Input: part model. Units: mm. Frame: model coordinates. A direction names the side the tool comes from. Give positions to 0.01 mm unless a question says otherwise; leave off trailing zeros. Order: outer loops, then holes, each group sorted by start corner. A loop starts at its lowest first (then second) coordinate and runs counter-clockwise, first axis right, second up. Notation, with made-up numbers: (62.5, 31) - (116.5, 31) arc R12 ccw to (116.5, 52) - close; hole circle Ø9 at (78.25, 5.25). An arc over 180 degrees is marked (long way). Answer in a Markdown table with one row per item. Add a question column.
1. Section query D-D on y = 48.5. Return loops of the section in (x, z).
2. Section query C-C on z = 0. Return loops of the section in (x, y).
3. Mould query, pull axis Y, two halves, no side actions, for faces 6 (the face through (15, 28, 15)), 7 (the face through (-15.25, 40, 0)), 8 (the face through (0, 25, 20.5)). Classes: released by +Y, released by -Y, zero draft, split by the parting line, or undercut.
4. Section query A-A on y = 26.5. Return loops of the section in (x, z), and give its area (3 significant figures).
5. Access query for faces 1 (the face through (-15, 28, -15)), 2 (the face through (0, 57, -22)), 3 (the face through (0, 58, -22)), 4 (the face through (-13.82, 40.14, -13.75)), 5 (the face through (0, 25, -20.5)). Directions: +Z, -Z, +X, -X, +Y, -Y. A direction counts if a zero-diameter tool reaches every point of the face in a straight line with its end or side. Return the directions, or none.
6. Ray query, line 1 (Z direction, x = -15.25, y = 23); line 2 (Y direction, x = -9, z = 17.5); line 3 (X direction, y = 32.25, z = 0). Return the intervals inside material, ascending. Write a range as [from, to].
7. Contact query for flat-ended pins moving along their axis: pin 1 (8 mm diameter, centred on x = 2, z = 13, fed in from -Y); pin 2 (4 mm diameter, centred on x = 15.25, z = -15.25, fed in from -Y); pin 3 (5 mm diameter, centred on y = 9, z = 0, fed in from -X). Output: stop coordinate, or through.
```python
from build123d import *

# Parameters (mm, degrees)
SKETCH1_R           = 2.5
BOSS_EXTRUDE1_DEPTH = 20
BOSS_EXTRUDE2_START = 20
SKETCH1_3_W         = 41
SKETCH1_3_H         = 41
SKETCH1_3_W_2       = 30.5
SKETCH1_3_H_2       = 30.5
SKETCH1_3_R         = 2.5
BOSS_EXTRUDE2_DEPTH = 10
BOSS_EXTRUDE3_START = 20
SKETCH1_4_W         = 30.5
SKETCH1_4_H         = 30.5
SKETCH1_4_R         = 2.5
BOSS_EXTRUDE3_DEPTH = 30
BOSS_EXTRUDE4_START = 50
SKETCH1_5_W         = 41
SKETCH1_5_H         = 41
BOSS_EXTRUDE4_DEPTH = 10
FILLET1_R           = 5
SKETCH2_R           = 1.75
CUT_EXTRUDE1_DEPTH  = 8
SKETCH3_R           = 13
BOSS_EXTRUDE5_DEPTH = 4
CHAMFER1_SIZE       = 1
SKETCH4_W           = 17
SKETCH4_H           = 6
SKETCH4_W_2         = 15
SKETCH4_H_2         = 4
EXTRUDE_THIN1_DEPTH = 3


with BuildPart() as part:
    # Sketch1 → Boss-Extrude1 (new body)
    with BuildSketch(Plane(origin=(0, 0, 0), x_dir=(1, 0, 0), z_dir=(0, 1, 0))):
        Circle(SKETCH1_R)
    extrude(amount=BOSS_EXTRUDE1_DEPTH)



with BuildPart() as body_2:
    # Sketch1_3 → Boss-Extrude2 (new body)
    with BuildSketch(Plane(origin=(0, 0, 0), x_dir=(1, 0, 0), z_dir=(0, 1, 0)).offset(BOSS_EXTRUDE2_START)):
        Rectangle(SKETCH1_3_W, SKETCH1_3_H)
        Rectangle(SKETCH1_3_W_2, SKETCH1_3_H_2, mode=Mode.SUBTRACT)
        Rectangle(SKETCH1_3_W_2, SKETCH1_3_H_2)
        Circle(SKETCH1_3_R, mode=Mode.SUBTRACT)
    extrude(amount=BOSS_EXTRUDE2_DEPTH)

    # Sketch1_4 → Boss-Extrude3 (add)
    with BuildSketch(Plane(origin=(0, 0, 0), x_dir=(1, 0, 0), z_dir=(0, 1, 0)).offset(BOSS_EXTRUDE3_START)):
        Rectangle(SKETCH1_4_W, SKETCH1_4_H)
        Circle(SKETCH1_4_R, mode=Mode.SUBTRACT)
    extrude(amount=BOSS_EXTRUDE3_DEPTH)

    # Sketch1_5 → Boss-Extrude4 (add)
    with BuildSketch(Plane(origin=(0, 0, 0), x_dir=(1, 0, 0), z_dir=(0, 1, 0)).offset(BOSS_EXTRUDE4_START)):
        Rectangle(SKETCH1_5_W, SKETCH1_5_H)
    extrude(amount=BOSS_EXTRUDE4_DEPTH)

    # Fillet1
    fillet1_edges = [body_2.edges().sort_by_distance(p)[0] for p in [
        (-20.5, 25, -20.5),
        (20.5, 25, -20.5),
        (20.5, 25, 20.5),
        (-20.5, 25, 20.5),
        (-15.25, 40, -15.25),
        (-15.25, 40, 15.25),
        (15.25, 40, 15.25),
        (15.25, 40, -15.25),
        (20.5, 55, 20.5),
        (20.5, 55, -20.5),
        (-20.5, 55, -20.5),
        (-20.5, 55, 20.5),
    ]]
    fillet(fillet1_edges, radius=FILLET1_R)

    # Sketch2 → Cut-Extrude1 (cut)
    with BuildSketch(Plane.XZ.offset(-20)):
        with Locations((15.25, -15.25)):
            Circle(SKETCH2_R)
        with Locations((-15.25, -15.25)):
            Circle(SKETCH2_R)
    cut_extrude1 = extrude(amount=-CUT_EXTRUDE1_DEPTH, mode=Mode.SUBTRACT)

    # Mirror1: Cut-Extrude1 across plane
    add(cut_extrude1.mirror(Plane.XY), mode=Mode.SUBTRACT)


with BuildPart() as part_1:
    add(part.part)

    add(body_2.part)  # Boss-Extrude5 merges body 2
    # Sketch3 → Boss-Extrude5 (add)
    with BuildSketch(Plane.XZ.offset(-20)):
        Circle(SKETCH3_R)
    extrude(amount=BOSS_EXTRUDE5_DEPTH)

    # Chamfer1
    chamfer1_edges = [part_1.edges().sort_by_distance(p)[0] for p in [
        (-13, 16, 0),
    ]]
    chamfer(chamfer1_edges, length=CHAMFER1_SIZE)

    # Sketch4 → Extrude-Thin1 (add)
    with BuildSketch(Plane.XY.offset(-20.5)):
        with Locations((0, 55)):
            Rectangle(SKETCH4_W, SKETCH4_H)
        with Locations((0, 55)):
            Rectangle(SKETCH4_W_2, SKETCH4_H_2, mode=Mode.SUBTRACT)
    extrude(amount=-EXTRUDE_THIN1_DEPTH)


solid = part_1.part
```
Answer:
| question | item | result |
|---|---|---|
| 1 | outline | (-15.25, -10.25) arc R5 ccw to (-10.25, -15.25) - (10.25, -15.25) arc R5 ccw to (15.25, -10.25) - (15.25, 10.25) arc R5 ccw to (10.25, 15.25) - (-10.25, 15.25) arc R5 ccw to (-15.25, 10.25) - close; hole circle Ø5 at (0, 0) |
| 2 | outline | (-20.5, 20) - (-13, 20) - (-13, 17) - (-12, 16) - (-2.5, 16) - (-2.5, 0) - (2.5, 0) - (2.5, 16) - (12, 16) - (13, 17) - (13, 20) - (20.5, 20) - (20.5, 30) - (15.25, 30) - (15.25, 50) - (20.5, 50) - (20.5, 60) - (-20.5, 60) - (-20.5, 50) - (-15.25, 50) - (-15.25, 30) - (-20.5, 30) - close; hole (-2.5, 20) - (2.5, 20) - (2.5, 50) - (-2.5, 50) - close |
| 3 | face 6 | released by -Y |
| 3 | face 7 | undercut |
| 3 | face 8 | zero draft |
| 4 | outline | (-20.5, -15.5) arc R5 ccw to (-15.5, -20.5) - (15.5, -20.5) arc R5 ccw to (20.5, -15.5) - (20.5, 15.5) arc R5 ccw to (15.5, 20.5) - (-15.5, 20.5) arc R5 ccw to (-20.5, 15.5) - close; hole circle Ø3.5 at (-15.25, -15.25); hole circle Ø3.5 at (-15.25, 15.25); hole circle Ø5 at (0, 0); hole circle Ø3.5 at (15.25, -15.25); hole circle Ø3.5 at (15.25, 15.25) |
| 4 | area | 1,600 mm² |
| 5 | face 1 | -Y |
| 5 | face 2 | -Z |
| 5 | face 3 | -Z, +X, -X, +Y |
| 5 | face 4 | -Z, -X |
| 5 | face 5 | -Z, +X, -X, -Y |
| 6 | line 1 | z = [-20.5, -17], [-13.5, 13.5], [17, 20.5] |
| 6 | line 2 | y = [20, 30], [50, 60] |
| 6 | line 3 | x = [-15.25, -2.5], [2.5, 15.25] |
| 7 | pin 1 | stops at y = 16 |
| 7 | pin 2 | stops at y = 20 |
| 7 | pin 3 | stops at x = -2.5 |
